Drawing for the job (mm, zero at the part's lowest x, y, z). Round coordinates to 2 decimals unless told otherwise and drop trailing zeros. Order: outer loops, then holes, each group sorted by start corner. A loop starts at its lowest first (then second) coordinate and runs counter-clockwise, first axis right, second up. Notation, with made-up numbers: (83.25, 39) - (135.25, 39) arc R33 cw to (135.25, 73) - close; hole circle Ø1 at (4, -30). An arc over 180 degrees is marked (long way). Answer as a JSON object with one key per item and string values.
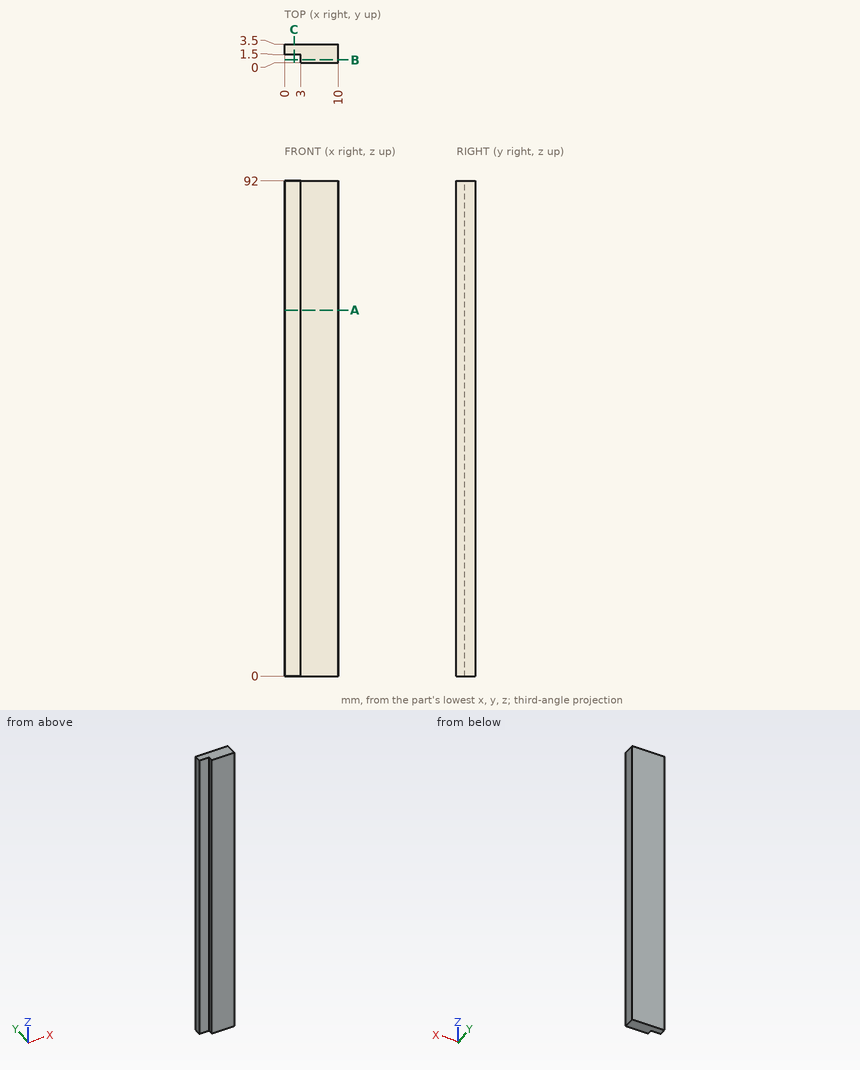
Item 1: Cut at B-B (y = 0.55). Write the cut outline in (x, z).
Taken from the geometry:
{"outline": "(3, 0) - (10, 0) - (10, 92) - (3, 92) - close"}
Item 2: Cut at A-A (z = 68). Write the cut outline in (x, y), plus the area to 3 significant figures.
Taken from the geometry:
{"outline": "(0, 1.5) - (3, 1.5) - (3, 0) - (10, 0) - (10, 3.5) - (0, 3.5) - close", "area": "30.5 mm2"}
Item 3: Probe L1, parallel to X at y = 0.45, z = 56; L2, parallel to Y at x = 1.25, z = 66. List the from-to ranges inside material, lowest first. Write a range as from..to.
Taken from the geometry:
{"L1": "3..10", "L2": "1.5..3.5"}
Item 4: Cut at C-C (x = 1.75). Write the cut outline in (y, z).
Taken from the geometry:
{"outline": "(1.5, 0) - (3.5, 0) - (3.5, 92) - (1.5, 92) - close"}
Item 5: Drop flat-ended pins along their axis: P1, Ø1.6, axis at y = 0.5, z = 32, coming from the -X side; P2, Ø0.9, axis at x = 2, z = 26, coming from the -Y side. Give the stop position or say it passes through.
Taken from the geometry:
{"P1": "x = 3", "P2": "y = 1.5"}
